from build123d import *

# Parameters (mm, degrees)
ESQUISSE1_W                = 614.6
ESQUISSE1_H                = 372.95
BOSS_EXTRU_1_DEPTH         = 3.175
ENL_V_MAT_EXTRU_1_DEPTH    = 360.508745547
D_GAGEMENT_121_D           = 5.7912
R_P_TITION_LIN_AIRE1_COUNT = 3
R_P_TITION_LIN_AIRE1_PITCH = 150
ENL_V_MAT_EXTRU_2_DEPTH    = 360.508745547
ESQUISSE10_W               = 1.35
ESQUISSE10_H               = 372.95
BOSS_EXTRU_3_DEPTH         = 6.35
D_GAGEMENT_61_D            = 4.3053


with BuildPart() as part:
    # Esquisse1 → Boss.-Extru.1 (new, symmetric)
    with BuildSketch(Plane.XY):
        Rectangle(ESQUISSE1_W, ESQUISSE1_H)
    extrude(amount=BOSS_EXTRU_1_DEPTH, both=True)

    # Esquisse2 → Enlèv. mat.-Extru.1 (cut, through all)
    with BuildSketch(Plane.XY.offset(3.175)):
        with BuildLine():
            Line((-22.3, 17.475), (-22.3, -62.525))
            ThreePointArc((-22.3, -62.525), (-82.3, -122.525), (-142.3, -62.525))
            Line((-142.3, -62.525), (-142.3, 17.475))
            ThreePointArc((-142.3, 17.475), (-82.3, 77.475), (-22.3, 17.475))
        make_face()
    enl_v_mat_extru_1 = extrude(amount=-ENL_V_MAT_EXTRU_1_DEPTH, mode=Mode.SUBTRACT)

    # Dégagement #121 (through all)
    with Locations(Plane.XY.offset(3.175)):
        with Locations((-127.3, -114.831787322), (-37.3, -114.831787322), (-37.3, 69.781787322), (-127.3, 69.781787322)):
            d_gagement_121 = Hole(D_GAGEMENT_121_D / 2)

    # Répétition linéaire1: Enlèv. mat.-Extru.1, Dégagement #121 ×3
    with Locations(*[(i * R_P_TITION_LIN_AIRE1_PITCH, 0, 0) for i in range(1, R_P_TITION_LIN_AIRE1_COUNT)]):
        add(enl_v_mat_extru_1, mode=Mode.SUBTRACT)
        add(d_gagement_121, mode=Mode.SUBTRACT)

    # Esquisse9 → Enlèv. mat.-Extru.2 (cut, through all)
    with BuildSketch(Plane(origin=(0, 0, -3.175), x_dir=(-1, 0, 0), z_dir=(0, 0, -1))):
        Polygon((247.301989616, 186.475), (307.3, 126.476989616), (307.3, 186.475), align=None)
    enl_v_mat_extru_2 = extrude(amount=-ENL_V_MAT_EXTRU_2_DEPTH, mode=Mode.SUBTRACT)

    # Esquisse10 → Boss.-Extru.3 (add, through all)
    with BuildSketch(Plane.XY.offset(3.175)):
        with Locations((307.975, 0)):
            Rectangle(ESQUISSE10_W, ESQUISSE10_H)
    extrude(amount=-BOSS_EXTRU_3_DEPTH)

    # Dégagement #61 (through all)
    with Locations(Plane(origin=(0, 0, -3.175), x_dir=(-1, 0, 0), z_dir=(0, 0, -1))):
        with Locations((276.225000899, -77.375), (196.850000899, -156.075), (-16.549999101, -156.075), (-229.949999101, -156.075), (-229.949999101, 156.075), (-16.549999101, 156.075), (196.850000899, 156.075), (276.225000899, 77.375)):
            Hole(D_GAGEMENT_61_D / 2)

    # Symétrie1: Enlèv. mat.-Extru.2 across plane
    add(enl_v_mat_extru_2.mirror(Plane.ZX), mode=Mode.SUBTRACT)


solid = part.part
Can you work these out from the model? Positions are in its coordinate system, mm. A direction names the side the tool comes from. Coordinates: 2 decimals unless noted, no trailing zeros. Order: outer loops, then holes, each group sorted by start corner. A loop starts at its lowest first (then second) coordinate and runs counter-clockwise, first axis right, second up. Notation, with made-up numbers: (-3.5, 34.25) -> (44.5, 34.25) arc R18 cw to (44.5, 58.25) -> close; hole circle Ø8 at (9.25, 12.5). An arc over 180 degrees is marked (long way). Use one line per item in the form item = value.
Q1. Imagine slicing it at A-A, the plane x = -82.3. List the corners of the cut face in (y, z) for me (3 decimals), then the cut area to 3 significant figures.
From the geometry:
outline = (-186.475, -3.175) -> (-122.525, -3.175) -> (-122.525, 3.175) -> (-186.475, 3.175) -> close; (77.475, -3.175) -> (186.475, -3.175) -> (186.475, 3.175) -> (77.475, 3.175) -> close
area = 1,100 mm²
Q2. Imagine slicing it at C-C, the plane z = 1.5. Give the number of separate pieces and of enclosed holes in the cut face, then the cut area to 3 significant figures.
From the geometry:
separate_pieces = 1
enclosed_holes = 23
area = 163,000 mm²
Q3. Will these pins go through, and if not, where does the flat tip stop? P1, Ø5, axis at x = 16.55, y = 156.075, coming from the -Z side (3 decimals); P2, Ø3.5, axis at x = 229.95, y = 156.075, coming from the +Z side.
From the geometry:
P1 = -3.175
P2 = through
Q4. I need wall thicknesses on L1, parallel to X at y = -9, z = 2; L2, parallel to Y at x = 172.7, z = 1.5 (3 decimals); L3, parallel to X at y = -79, z = -2.25. Which ranges of each line are inside material? Lowest first, please.
From the geometry:
L1 = -307.3 to -142.3, -22.3 to 7.7, 127.7 to 157.7, 277.7 to 308.65
L2 = -186.475 to -117.727, -111.936 to -102.211, 57.161 to 66.886, 72.677 to 186.475
L3 = -307.3 to -277.64, -274.81 to -139.99, -24.61 to 10.01, 125.39 to 160.01, 275.39 to 308.65
Q5. Which directions (+Z, -Z, +X, -X, +Y, -Y) give clear straight access to the entire face, cutting with the end or side of a thin tool? Please do faces 1 (the face through (69.02, -122.51, 0.04)), 2 (the face through (-4, 3, 3.175)).
From the geometry:
face_1 = +Z, -Z
face_2 = +Z, +X, -X, +Y, -Y
Q6. Imagine slicing it at B-B, the plane x = 216. List the corners of the cut face in (y, z) for me (3 decimals), then the cut area to 3 significant figures.
From the geometry:
outline = (-186.475, -3.175) -> (-122.501, -3.175) -> (-122.501, 3.175) -> (-186.475, 3.175) -> close; (77.451, -3.175) -> (186.475, -3.175) -> (186.475, 3.175) -> (77.451, 3.175) -> close
area = 1,100 mm²
